```python
from build123d import *

# Parameters (mm, degrees)
F1_DEPTH = 6
F2_W     = 14.4
F2_H     = 4.4
F5_W     = 13.4
F5_H     = 3.4
F9_DEPTH = 4
F10_R    = 0.5


with BuildPart() as f1:
    # F0 (on Top) → F1 (new body)
    with BuildSketch(Plane.XY):
        Polygon((0, 2.8761399509), (0.5, 2.8761399509), (13.9, 2.8761399509), (14.4, 2.8761399509), (14.4, 3.3761399509), (0, 3.3761399509), align=None)
        Polygon((0, 10.3761399509), (0, 3.3761399509), (14.4, 3.3761399509), (14.4, 10.3761399509), (14.4, 11.8761399509), (12.9, 11.8761399509), (1.5, 11.8761399509), (0, 11.8761399509), align=None)
        with BuildLine():
            ThreePointArc((3, 9.3761399509), (3.2928932188, 10.0832467321), (4, 10.3761399509))
            Line((4, 10.3761399509), (10.4, 10.3761399509))
            ThreePointArc((10.4, 10.3761399509), (11.1071067812, 10.0832467321), (11.4, 9.3761399509))
            Line((11.4, 9.3761399509), (11.4, 8.5761399509))
            ThreePointArc((11.4, 8.5761399509), (11.1071067812, 7.8690331698), (10.4, 7.5761399509))
            Line((10.4, 7.5761399509), (4, 7.5761399509))
            ThreePointArc((4, 7.5761399509), (3.2928932188, 7.8690331698), (3, 8.5761399509))
            Line((3, 8.5761399509), (3, 9.3761399509))
        make_face(mode=Mode.SUBTRACT)
    extrude(amount=F1_DEPTH)

    # F4: sweep along a path in F3
    with BuildLine(Plane(origin=(0, 0, 0), x_dir=(0, -1, 0), z_dir=(-1, 0, 0))) as f4_path:
        Line((-2.8761399509, 0), (0.418709749, 9.4416082028))
    # F2 (on face) → F4 (sweep)
    with BuildSketch(Plane(origin=(0, 0, 0), x_dir=(1, 0, 0), z_dir=(0, 0, -1))):
        with Locations((7.2, -5.0770884661)):
            Rectangle(F2_W, F2_H)
    sweep(path=f4_path.line)

    # F7: sweep along a path in F6
    with BuildLine(Plane.YZ) as f7_path:
        Line((3.6174104522, 8.9695277927), (6.7475176671, 0))
    # F5 (on face) → F7 (sweep, cut)
    with BuildSketch(Plane(origin=(0, 0, 0), x_dir=(1, 0, 0), z_dir=(0, 0, -1))):
        with Locations((7.2, -5.0761399509)):
            Rectangle(F5_W, F5_H)
    sweep(path=f7_path.line, mode=Mode.SUBTRACT)

    # F8 (on Top) → F9 (cut)
    with BuildSketch(Plane.XY):
        Polygon((13.9, 11.3761399509), (12.4, 11.3761399509), (2, 11.3761399509), (0.5, 11.3761399509), (0.5, 9.8761399509), (0.5, 4.8761399509), (0.5, 3.3786750864), (2, 3.3761399509), (12.4, 3.3761399509), (13.9, 3.3761399509), (13.9, 4.8761399509), (13.9, 9.8761399509), align=None)
    extrude(amount=F9_DEPTH, mode=Mode.SUBTRACT)

    # F10
    f10_edges = [f1.edges().sort_by_distance(p)[0] for p in [
        (0, 1.782239, 9.441608),
        (7.2, 3.982239, 9.441608),
        (14.4, 1.782239, 9.441608),
        (7.2, -0.417761, 9.441608),
        (14.4, 11.87614, 3),
        (0, 11.87614, 3),
        (0.5, 11.37614, 2),
        (13.9, 11.37614, 2),
        (0.5, 1.811086, 4.484764),
        (13.9, 1.811086, 4.484764),
        (0, 4.58275, 7.720804),
        (0, 1.229189, 4.722163),
        (14.4, 4.58275, 7.720804),
        (0.5, 1.946033, 8.969528),
        (7.2, 0.246033, 8.969528),
        (7.2, 3.646033, 8.969528),
        (13.9, 1.946033, 8.969528),
        (14.4, 1.229189, 4.722163),
    ]]
    fillet(f10_edges, radius=F10_R)


solid = f1.part
```
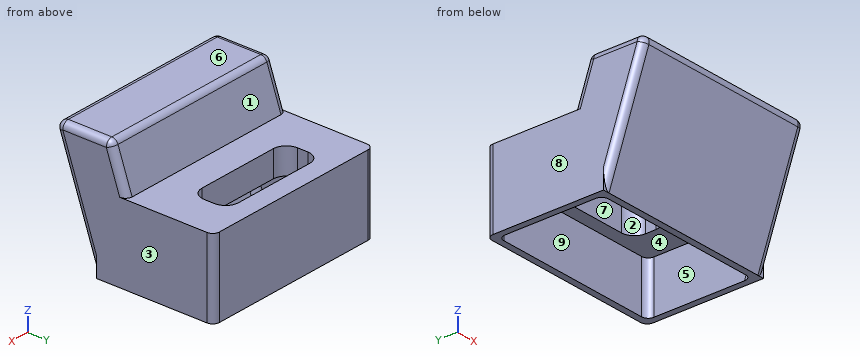
Verification items for the finished model (mm, model axes). Face numbers are marked on the shaded views. A direction names the side the tool comes from. Coordinates: 2 decimals unless noted, no trailing zeros. Write each loop counter-clockwise with the first axis right and the second up, starting at its lowest first coordinate (ties: lowest second). Pieces come first, ordered by that corner, then holes. Notation, with made-up numbers: M -0.75,5.5 L 8.25,5.5 A17 ccw 8.25,15.5 Z; hole C 67,45 d9. An arc over 180 degrees is marked long. Answer as a JSON object with one key per item and string values. Group by question number.
(1) Cross-section at B-B, the plane y = 8.25. Record the cut outline in (x, z), and give its area (3 significant figures).
(2) Release check for a two-part mould opening along X. For the marked faces 6, 7, 8 and 9 record: +X half, -X half, draft (parallel to the pull), parting line (faces both ways), or undercut.
(3) Cross-section at D-D, the plane z = 4.5. State how many separate pieces and enclosed holes the cut face has, and give its area (3 significant figures).
(4) Gauge pin test, flat ends, axial feed: pin 1 (2 mm diameter, centred on x = 7.5, z = 2.5, fed in from -Y); pin 2 (1.7 mm diameter, centred on x = 10, z = 0.5, fed in from -Y); pin 3 (1 mm diameter, centred on x = 2, y = 7.5, fed in from -Z). Record the tip position at first contact, or that the pin passes through.
(5) Tool access check on the marked faces 1, 2, 3, 4 and 5. Record the directions out of +Z, -Z, +X, -X, +Y, -Y that give a thin tool (end or side, any length) a straight path to the whole face; none if there is none.
(6) Material ranges on line 1 (X direction, y = 3, z = 2.5); line 2 (Z direction, x = 6.75, y = 7); line 3 (Y direction, x = 3, z = 7.5), recorded low to high.
Reply:
{
 "1": {"outline": "M 0,0 L 0.5,0 L 0.5,4 L 3.05,4 L 3.05,6 L 0,6 Z; M 11.35,4 L 13.9,4 L 13.9,0 L 14.4,0 L 14.4,6 L 11.35,6 Z", "area": "16.2 mm²"},
 "2": {"face 6": "draft", "face 7": "undercut", "face 8": "-X half", "face 9": "undercut"},
 "3": {"separate pieces": "1", "enclosed holes": "2", "area": "83.9 mm²"},
 "4": {"pin 1": "y = 1.66", "pin 2": "y = 2.41", "pin 3": "z = 4"},
 "5": {"face 1": "+Z, +X, -X, +Y", "face 2": "+Z, -Z", "face 3": "+Z, -Z, +X, +Y, -Y", "face 4": "-Z", "face 5": "none"},
 "6": {"line 1": "0 to 0.5, 13.9 to 14.4", "line 2": "4 to 6", "line 3": "0.26 to 0.76, 4.16 to 4.66"}
}
